Autodesk Inventor part; units mm, degrees
ref_plane "YZ Plane" through (0, 0, 0) normal (1, 0, 0) x (0, 1, 0)
ref_plane "XZ Plane" through (0, 0, 0) normal (0, 1, 0) x (-1, 0, 0)
ref_plane "XY Plane" through (0, 0, 0) normal (0, 0, 1) x (1, 0, 0)
sketch "スケッチ1" plane through (0, 0, 0) normal (0, 0, 1) x (1, 0, 0)
  circle A0 centre (0, 0) radius 40.5
  circle A1 centre (0, 440) radius 40.5
  line L0 (-40.5, 0) -> (-40.5, 440)
  line L1 (40.5, 440) -> (40.5, 0)
  dimension "d0" = 81
  dimension "d1" = 81
  dimension "d2" = 440
extrude "プレート1" add sketch "スケッチ1" along normal blind 2
sketch "スケッチ6" plane through (0, 0, 2) normal (0, 0, 1) x (1, 0, 0)
  arc A0 (40.5, 440) -> (-40.5, 440) centre (0, 440) ccw
  circle A1 centre (0, 440) radius 32.5
  point P0 (0, 0)
  dimension "d43" = 65
extrude "押し出し2" cut sketch "スケッチ6" against normal blind 10
sketch "スケッチ7" plane through (0, 0, 2) normal (0, 0, 1) x (1, 0, 0)
  arc A0 (40.5, 440) -> (-40.5, 440) centre (0, 440) ccw
  circle A1 centre (0, 440) radius 36.5
  point P0 (0, 0)
  point P1 (0, 476.5)
  point P2 (-31.6099, 458.25)
  point P3 (-31.6099, 421.75)
  point P4 (0, 403.5)
  point P5 (31.6099, 421.75)
  point P6 (31.6099, 458.25)
  dimension "d46" = 73
  dimension "d49" = 360
hole "穴4" at (0, 476.5, 2) at (-31.6099, 458.25, 2) at (-31.6099, 421.75, 2) at (0, 403.5, 2) at (31.6099, 421.75, 2) at (31.6099, 458.25, 2) direction (0, 0, -1) diameter 3.2 end through all
sketch "スケッチ8" plane through (0, 0, 2) normal (0, 0, 1) x (1, 0, 0)
  arc A0 (40.5, 440) -> (-40.5, 440) centre (0, 440) ccw
  circle A1 centre (0, 440) radius 25
  line L0 (23.4923, 431.4495) -> (-32.7335, 276.9703)
  line L1 (-23.4923, 448.5505) -> (-36.9957, 411.4503)
  line L2 (0, 603.9) -> (0, -147.9)
  circle A2 centre (0, 355.2097) radius 4
  point P0 (0, 0)
  point P1 (4, 72)
  dimension "d92" = 50
  dimension "d93" = 20
  dimension "d94" = 8
  dimension "d102" = 0
  dimension "d140" = 72
  dimension "d141" = 4
hole "穴5" at (4, 72, 2) at (0, 355.2097, 2) direction (0, 0, -1) diameter 4.3 end through all
sketch "スケッチ9" plane through (0, 0, 2) normal (0, 0, 1) x (1, 0, 0)
  circle A0 centre (0, 0) radius 67.5
  circle A1 centre (9, 84) radius 8
  arc A2 (40.5, 440) -> (-40.5, 440) centre (0, 440) ccw
  dimension "d69" = 84
  dimension "d79" = 135
  dimension "d80" = 16
  dimension "d144" = 9
hole "穴6" at (9, 84, 2) direction (0, 0, -1) diameter 4.3 end through all
sketch "スケッチ13" plane through (0, 0, 2) normal (0, 0, 1) x (1, 0, 0)
  circle A0 centre (0, 0) radius 15
  point P0 (0, 15)
  point P1 (-12.9904, 7.5)
  point P2 (-12.9904, -7.5)
  point P3 (0, -15)
  point P4 (12.9904, -7.5)
  point P5 (12.9904, 7.5)
  dimension "d109" = 30
  dimension "d112" = 360
hole "穴8" at (0, 15, 2) at (-12.9904, 7.5, 2) at (-12.9904, -7.5, 2) at (0, -15, 2) at (12.9904, -7.5, 2) at (12.9904, 7.5, 2) direction (0, 0, -1) diameter 3.4 end through all
sketch "スケッチ14" plane through (0, 0, 2) normal (0, 0, 1) x (1, 0, 0)
  circle A0 centre (0, 0) radius 10
  dimension "d121" = 20
extrude "押し出し5" cut sketch "スケッチ14" against normal blind 10
sketch "スケッチ15" plane through (0, 0, 2) normal (0, 0, 1) x (1, 0, 0)
  line L0 (-16, 84) -> (9, 84) construction
  line L1 (-16, 81.85) -> (9, 81.85)
  line L2 (9, 86.15) -> (-16, 86.15)
  arc A0 (-16, 86.15) -> (-16, 81.85) centre (-16, 84) ccw
  arc A1 (9, 81.85) -> (9, 86.15) centre (9, 84) ccw
  circle A2 centre (9, 84) radius 2.15
  point P0 (0, 0)
  dimension "d142" = 25
extrude "押し出し6" cut sketch "スケッチ15" against normal blind 10
sketch "スケッチ17" plane through (0, 0, 0) normal (0, 0, -1) x (-1, 0, 0)
  point P0 (0, 0)
  point P1 (0, 220)
  dimension "d132" = 220
hole "穴9" at (0, 220, 0) direction (0, 0, 1) diameter 4.5 end through all
sketch "スケッチ16" plane through (0, 0, 2) normal (0, 0, 1) x (1, 0, 0)
  line L0 (-21, 72) -> (4, 72) construction
  line L1 (-21, 69.85) -> (4, 69.85)
  line L2 (4, 74.15) -> (-21, 74.15)
  arc A0 (-21, 74.15) -> (-21, 69.85) centre (-21, 72) ccw
  arc A1 (4, 69.85) -> (4, 74.15) centre (4, 72) ccw
  circle A2 centre (4, 72) radius 2.15
  point P0 (0, 0)
  point P1 (-8.5, 72)
  dimension "d143" = 21
extrude "押し出し7" cut sketch "スケッチ16" against normal blind 10
equation "\"d56\" = Thickness"
equation "\"d67\" = Thickness"
equation "\"d77\" = Thickness"
equation "\"d119\" = Thickness"
equation "\"d138\" = Thickness"
equation "\"d3\" = Thickness"
equation "\"BendRadius\" = Thickness"
equation "\"BendReliefWidth\" = Thickness"
equation "\"BendReliefDepth\" = 0.5 * Thickness"
equation "\"CornerReliefSize\" = 4 * Thickness"
equation "\"MinimumRemnant\" = 2 * Thickness"
equation "\"TransitionRadius\" = BendRadius"
equation "\"JacobiRadiusSize\" = Thickness"
equation "\"GapSize\" = Thickness"
properties part number "link2-plate1" material "CFRP"
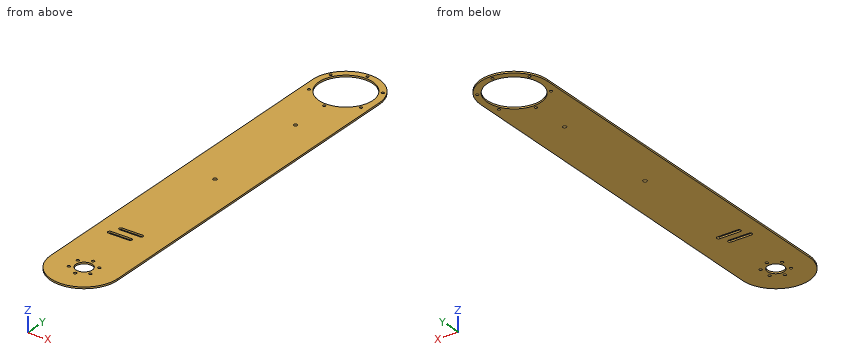
Can you work these out from the model? Positions are in its coordinate system, mm. Round coordinates to 2 decimals unless told otherwise and drop trailing zeros. Loops run counter-clockwise (first coordinate to the right, second up) from the corner with the lowest first, then second, coordinate; pieces in that order, holes last. Notation, with made-up numbers: (-8, -11) - (8, -11) arc R11 ccw to (8, 10) - close; hole circle Ø5 at (77, 35.5). An arc over 180 degrees is marked (long way). Write item = value, one per line. Start each with the question number.
(1) If we section it at B-B (x = 23): Please give me the cut outline in (y, z).
(2) If we section it at A-A (z = 1.35): Give the number of separate pieces and of enclosed holes in the cut face, and give its area (3 significant figures).
(3) For P1, Ø0.6, axis at x = -7.5, z = 1.5, coming from the -Y side, with a flat end and sliding along its axis, tell me the tip position at first contact or that it passes through.
(4) If I drill on probe 1 along Y at (x, z) = (-17.5, 0.8); probe 2 along Y at (x, z) = (3.5, 1.3); probe 3 along Y at (x, z) = (-33, 1.05), over which ranges is the centre line in solid material (lowest first)? Write a range as [from, to].
Ans:
q1.outline = (-33.34, 0) - (417.04, 0) - (417.04, 2) - (-33.34, 2) - close; (462.96, 0) - (473.34, 0) - (473.34, 2) - (462.96, 2) - close
q2.separate_pieces = 1
q2.enclosed_holes = 18
q2.area = 36,800 mm²
q3.P1 = -39.85
q4.probe_1 = [-36.52, 69.85], [74.15, 82.46], [85.54, 412.61], [467.39, 476.52]
q4.probe_2 = [-40.35, -9.37], [9.37, 69.85], [74.15, 81.85], [86.15, 407.69], [472.31, 480.35]
q4.probe_3 = [-23.48, 420.96], [422.54, 457.46], [459.04, 463.48]
